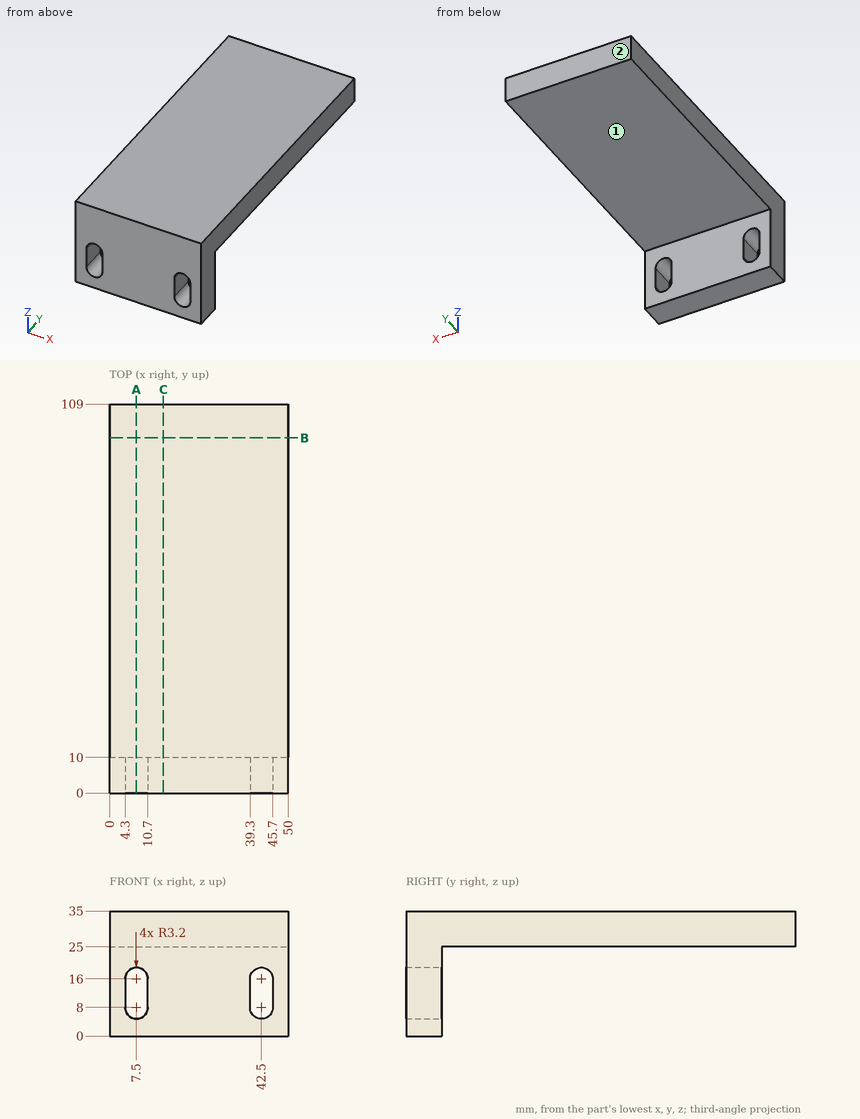
Source: three-view drawing plus pictorial views. Frame: mm from the lowest corner of the part. A direction names the side the tool comes from. Round coordinates to 2 decimals unless told otherwise and drop trailing zeros. Loops run counter-clockwise (first coordinate to the right, second up) from the corner with the lowest first, then second, coordinate; pieces in that order, holes last. Notation, with made-up numbers: M 68,29 L 123,29 A31 cw 123,53 Z; hole C -25,23 d5. An arc over 180 degrees is marked long. Put each result on its own line as item: value. Start each with the question number.
(1) Section query C-C (x = 15). Return loops of the section in (y, z).
(2) Section query B-B (y = 99.5). Return loops of the section in (x, z), then the cut area to 3 significant figures.
(3) Section query A-A (x = 7.5). Return loops of the section in (y, z).
(4) Material intervals for line 1 along Y through (x, z) = (17, 23); line 2 along Z through (x, y) = (5.5, 61.5), sorted ascending. Write a range as [from, to].
(5) Set-up query: the marked faces 1 and 2. Return all of +Z, -Z, +X, -X, +Y, -Y with unobstructed straight access to the full face (end or side cutting, diameter ignored); none if empty.
(6) Contact query for flat-ended pins moving along their axis: pin 1 Ø9 at (y, z) = (4, 10.5) entering from -X; pin 2 Ø12.5 at (x, z) = (29.5, 14.5) entering from +Y; pin 3 Ø5 at (y, z) = (57.5, 21) entering from +X; pin 4 Ø1.5 at (x, y) = (28, 11.5) entering from -Z. Output: stop coordinate, or through.
Findings below:
1. outline: M 0,0 L 10,0 L 10,25 L 109,25 L 109,35 L 0,35 Z
2. outline: M 0,25 L 50,25 L 50,35 L 0,35 Z
2. area: 500 mm2
3. outline: M 0,0 L 10,0 L 10,4.8 L 0,4.8 Z; M 0,19.2 L 10,19.2 L 10,25 L 109,25 L 109,35 L 0,35 Z
4. line 1: y = [0, 10]
4. line 2: z = [25, 35]
5. face 1: -Z, +X, -X, +Y
5. face 2: +Z, -Z, +X, -X, +Y
6. pin 1: stops at x = 0
6. pin 2: stops at y = 10
6. pin 3: passes through
6. pin 4: stops at z = 25
